Source: CAD feature listing. Evaluate the final solid. Frame: model axes, mm. Face numbers are marked on the shaded views. A direction names the side the tool comes from. Give positions to 0.01 mm unless a question says otherwise; leave off trailing zeros. Order: outer loops, then holes, each group sorted by start corner. A loop starts at its lowest first (then second) coordinate and runs counter-clockwise, first axis right, second up.
1) Draft query along Z for the marked faces 4, 5 and 6. Return one class per face: released by +Z, released by -Z, zero draft, split by the parting line, or undercut.
2) Section A-A, the plane z = -5.5. Return loops of the section in (x, y).
3) Material intervals for line 1 (Z direction, x = 15.25, y = 8.5); line 2 (X direction, y = 3, z = -10); line 3 (X direction, y = 3.75, z = 11.25), sorted ascending.
4) Section C-C, the plane z = -10. Return loops of the section in (x, y).
5) Section D-D, the plane x = 14. Return loops of the section in (y, z), plus the area to 4 significant figures.
6) Access query for the marked faces 1, 2 and 3. Directions: +Z, -Z, +X, -X, +Y, -Y. A direction counts if a zero-diameter tool reaches every point of the face in a straight line with its end or side. Return the directions, or none.
7) Section B-B, the plane y = 9.5. Return loops of the section in (x, z).
8) First-contact query: P1, Ø4.5, axis at x = 23.5, z = 0, coming from the +Y side; P2, Ø3.5, axis at x = 25, z = -10, coming from the +Y side; P3, Ø4.5, axis at x = 18.5, y = 8.5, coming from the -Z side; P4, Ø3, axis at x = 21, y = 10, coming from the +Z side. Flat tips, straight axial feed; report the tip coordinate or a pass-through.
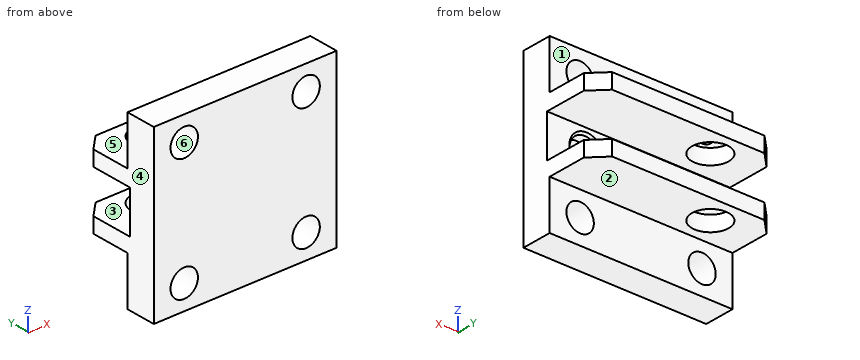
```python
from build123d import *

# Parameters (mm, degrees)
BOSS_EXTRUDE1_DEPTH      = 14
BOSS_EXTRUDE1_DEPTH_BACK = 14
CUT_EXTRUDE1_DEPTH       = 14
CUT_EXTRUDE1_DEPTH_BACK  = 14
SKETCH2_R                = 3
CUT_EXTRUDE2_DEPTH       = 3.5
CUT_EXTRUDE2_DEPTH_BACK  = 3.5
SKETCH3_W                = 30
SKETCH3_H                = 9.5
SKETCH5_W                = 56
SKETCH5_H                = 28
CUT_EXTRUDE3_DEPTH       = 30
SKETCH6_R                = 2.25
CUT_EXTRUDE4_DEPTH       = 5
SKETCH7_R                = 2.25
CUT_EXTRUDE5_DEPTH       = 5
SKETCH8_R                = 2.25
CUT_EXTRUDE6_DEPTH       = 5
SKETCH9_R                = 2.25
CUT_EXTRUDE7_DEPTH       = 5


with BuildPart() as part:
    # Sketch1 → Boss-Extrude1 (new, two sides: drawn at the far end of the back side and taken through both)
    with BuildSketch(Plane.XY.offset(-BOSS_EXTRUDE1_DEPTH_BACK)):
        Polygon((0, 11.5), (0, 0), (30, 0), (30, 11.5), (27.5, 14), (2.5, 14), align=None)
    extrude(amount=BOSS_EXTRUDE1_DEPTH + BOSS_EXTRUDE1_DEPTH_BACK)

    # Sketch2 → Cut-Extrude1 (cut, two sides: drawn at the far end of the back side and taken through both)
    with BuildSketch(Plane.XY.offset(-CUT_EXTRUDE1_DEPTH_BACK)):
        with Locations((7.5, 9.5)):
            Circle(SKETCH2_R)
    extrude(amount=CUT_EXTRUDE1_DEPTH + CUT_EXTRUDE1_DEPTH_BACK, mode=Mode.SUBTRACT)

    # Sketch3 → Cut-Extrude2 (cut, two sides: drawn at the far end of the back side and taken through both)
    with BuildSketch(Plane.XY.offset(-CUT_EXTRUDE2_DEPTH_BACK)):
        with Locations((15, 9.25)):
            Rectangle(SKETCH3_W, SKETCH3_H)
    extrude(amount=CUT_EXTRUDE2_DEPTH + CUT_EXTRUDE2_DEPTH_BACK, mode=Mode.SUBTRACT)

    # Sketch4 → Cut-Revolve1 (revolve, cut)
    with BuildSketch(Plane.XY, mode=Mode.PRIVATE) as cut_revolve1_sk:
        Polygon((23.5, 4.5), (26.353553391, 4.5), (26, 4.146446609), (26, 2.5), (23.5, 2.5), align=None)
    revolve(cut_revolve1_sk.sketch.rotate(Axis((23.5, 2.5, 0), (0, 1, 0)), 270), axis=Axis((23.5, 2.5, 0), (0, 1, 0)), mode=Mode.SUBTRACT)

    # Sketch5 → Cut-Extrude3 (cut)
    with BuildSketch(Plane(origin=(0, 0, 0), x_dir=(0, 0, -1), z_dir=(1, 0, 0))):
        with Locations((0, 12)):
            Rectangle(SKETCH5_W, SKETCH5_H)
        Polygon((-14, 5), (-14, 0), (14, 0), (14, 5), (6, 5), (6, 14), (-6, 14), (-6, 5), align=None, mode=Mode.SUBTRACT)
    extrude(amount=CUT_EXTRUDE3_DEPTH, mode=Mode.SUBTRACT)

    # Sketch6 → Cut-Extrude4 (cut)
    with BuildSketch(Plane(origin=(0, 0, 0), x_dir=(1, 0, 0), z_dir=(0, 1, 0))):
        with Locations(Location((5, -10, 0), (0, 0, 270))):
            Circle(SKETCH6_R)
    extrude(amount=CUT_EXTRUDE4_DEPTH, mode=Mode.SUBTRACT)

    # Sketch7 → Cut-Extrude5 (cut)
    with BuildSketch(Plane(origin=(0, 0, 0), x_dir=(1, 0, 0), z_dir=(0, 1, 0))):
        with Locations(Location((25, 10, 0), (0, 0, 270))):
            Circle(SKETCH7_R)
    extrude(amount=CUT_EXTRUDE5_DEPTH, mode=Mode.SUBTRACT)

    # Sketch8 → Cut-Extrude6 (cut)
    with BuildSketch(Plane(origin=(0, 0, 0), x_dir=(1, 0, 0), z_dir=(0, 1, 0))):
        with Locations(Location((25, -10, 0), (0, 0, 270))):
            Circle(SKETCH8_R)
    extrude(amount=CUT_EXTRUDE6_DEPTH, mode=Mode.SUBTRACT)

    # Sketch9 → Cut-Extrude7 (cut)
    with BuildSketch(Plane(origin=(0, 0, 0), x_dir=(1, 0, 0), z_dir=(0, 1, 0))):
        with Locations(Location((5, 10, 0), (0, 0, 270))):
            Circle(SKETCH9_R)
    extrude(amount=CUT_EXTRUDE7_DEPTH, mode=Mode.SUBTRACT)


solid = part.part
```
From the geometry:
1. face 4: zero draft
1. face 5: released by +Z
1. face 6: undercut
2. outline: (0, 0) - (30, 0) - (30, 11.5) - (27.5, 14) - (2.5, 14) - (0, 11.5) - close; hole circle Ø6 at (7.5, 9.5)
3. line 1: z = -6 to -3.5, 3.5 to 6
3. line 2: x = 0 to 2.75, 7.25 to 22.75, 27.25 to 30
3. line 3: x = 0 to 3.13, 6.87 to 23.13, 26.87 to 30
4. outline: (0, 0) - (2.75, 0) - (2.75, 5) - (0, 5) - close; (7.25, 0) - (22.75, 0) - (22.75, 5) - (7.25, 5) - close; (27.25, 0) - (30, 0) - (30, 5) - (27.25, 5) - close
5. outline: (0, -14) - (5, -14) - (5, -6) - (14, -6) - (14, -3.5) - (4.5, -3.5) - (4.5, 3.5) - (14, 3.5) - (14, 6) - (5, 6) - (5, 14) - (0, 14) - close
5. area: 181.5 mm2
6. face 1: +Z, +X, -X, +Y
6. face 2: -Z, +X, -X, +Y
6. face 3: +X, -X, +Y
7. outline: (0, -6) - (4.5, -6) - (4.5, -3.5) - (0, -3.5) - close; (0, 3.5) - (4.5, 3.5) - (4.5, 6) - (0, 6) - close; (10.5, -6) - (30, -6) - (30, -3.5) - (10.5, -3.5) - close; (10.5, 3.5) - (30, 3.5) - (30, 6) - (10.5, 6) - close
8. P1: stops at y = 2.5
8. P2: passes through
8. P3: stops at z = -6
8. P4: stops at z = 6
